Could you check a few things on this model? Use its own coordinates, in mm. A direction names the side the tool comes from. Give positions to 0.01 mm unless a question says otherwise; leave off trailing zeros. Order: outer loops, then holes, each group sorted by start corner. A loop starts at its lowest first (then second) coordinate and runs counter-clockwise, first axis right, second up. Notation, with made-up numbers: (44.25, -28) -> (96.25, -28) arc R29 cw to (96.25, 9) -> close; hole circle Ø10 at (-25.5, 55.5). An arc over 180 degrees is marked (long way). Answer as CSV lines item,"result". Start each with the question number.
(1) We'd pull the mould along X, two halves only. Please class faces 1 (the face through (-11.721, 22.534, 9.392)), 2 (the face through (0.52, -12.69, 9.39)), 3 (the face through (-5, -12, 19.05)): released by +X, released by -X, zero draft, split by the parting line, or undercut.
(2) I want a section at A-A (x = 0). Please give me the cut outline in (y, z), plus the area to 3 significant figures.
(3) Will these pins go through, and if not, where does the flat tip stop? pin 1 Ø1.2 at (y, z) = (14.5, 9) entering from -X; pin 2 Ø1 at (x, z) = (-15, 6.5) entering from +Y; pin 3 Ø2 at (y, z) = (13.5, 14) entering from +X.
(4) I want a section at D-D (x = 21.5). Please give me the cut outline in (y, z).
(5) I want a section at B-B (y = 0). Please give me the cut outline in (x, z).
(6) On a 3-axis mill with a long thin cutter (end or side, diameter ignored), from which of +Z, -Z, +X, -X, +Y, -Y can I reach the whole of each face in a straight line? I mean faces 4 (the face through (-5, -12, 0)), 5 (the face through (-2.54, 14, 9)). Say none if no direction works.
(7) I want a section at C-C (z = 14.5). Please give me the cut outline in (x, y).
(8) I need wall thicknesses on L1, parallel to Y at x = 0, z = 17; L2, parallel to Y at x = -7, z = 4.5; L3, parallel to X at y = 8.5, z = 14. Which ranges of each line are inside material? Lowest first, please.
```python
from build123d import *

# Parameters (mm, degrees)
SKETCH3_R           = 25.4
BOSS_EXTRUDE1_DEPTH = 19.05


with BuildPart() as part:
    # Sketch3 → Boss-Extrude1 (new body)
    with BuildSketch(Plane.XY):
        with Locations(Location((0, 0, 0), (0, 0, 180))):
            Circle(SKETCH3_R)
        with BuildLine():
            Line((-2.54, 16.51), (2.54, 16.51))
            Line((2.54, 16.51), (2.54, 12.443407893))
            ThreePointArc((2.54, 12.443407893), (0, -12.7), (-2.54, 12.443407893))
            Line((-2.54, 12.443407893), (-2.54, 16.51))
        make_face(mode=Mode.SUBTRACT)
    extrude(amount=BOSS_EXTRUDE1_DEPTH)


solid = part.part
```
Final values:
1,face 1,"split by the parting line"
1,face 2,"undercut"
1,face 3,"zero draft"
2,outline,"(-25.4, 0) -> (-12.7, 0) -> (-12.7, 19.05) -> (-25.4, 19.05) -> close; (16.51, 0) -> (25.4, 0) -> (25.4, 19.05) -> (16.51, 19.05) -> close"
2,area,"411 mm²"
3,pin 1,"x = -21.26"
3,pin 2,"y = 20.85"
3,pin 3,"x = 22.11"
4,outline,"(-13.52, 0) -> (13.52, 0) -> (13.52, 19.05) -> (-13.52, 19.05) -> close"
5,outline,"(-25.4, 0) -> (-12.7, 0) -> (-12.7, 19.05) -> (-25.4, 19.05) -> close; (12.7, 0) -> (25.4, 0) -> (25.4, 19.05) -> (12.7, 19.05) -> close"
6,face 4,"-Z, +X, -X, +Y, -Y"
6,face 5,"+Z, -Z"
7,outline,"circle Ø50.8 at (0, 0); hole (-2.54, 12.44) arc R12.7 ccw (long way) to (2.54, 12.44) -> (2.54, 16.51) -> (-2.54, 16.51) -> close"
8,L1,"-25.4 to -12.7, 16.51 to 25.4"
8,L2,"-24.42 to -10.6, 10.6 to 24.42"
8,L3,"-23.94 to -9.44, 9.44 to 23.94"
